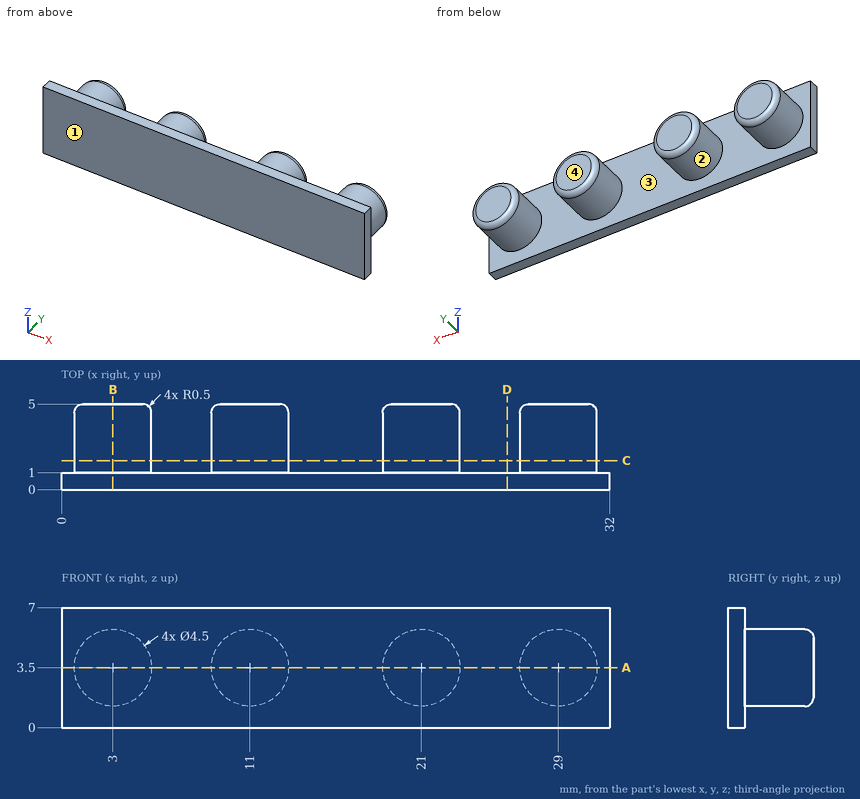
Answer from the drawing. Dimensions are ordinates in mm from the lowest x, y and z of the part. A direction names the side the tool comes from. Give positions to 0.01 mm unless a question says otherwise; leave off trailing zeros. Loops run counter-clockwise (first coordinate to the right, second up) from the corner with the lowest first, then second, coordinate; pieces in that order, holes last.
Item 1: Find the intervals of material crossed by line 1 along X through (y, z) = (2.4, 3.5); line 2 along X through (y, z) = (4.6, 5.5); line 3 along Y through (x, z) = (24, 4), in increasing order.
Item 2: The part is cut by section A-A (z = 3.5). Write down the section's boundary in (x, y), and give its area (3 significant figures).
Item 3: The part is cut by section C-C (y = 1.7). Write down the section's boundary in (x, z).
Item 4: Each of these flat-tipped pins is pushed along its axis until it touches: pin 1 Ø1.5 at (y, z) = (2.5, 2) entering from +X; pin 2 Ø1 at (y, z) = (3.5, 1) entering from +X. Where does it stop, or does it pass through?
Item 5: The mould has two halves that part along X. Classify the marked faces 3 and 4: released by +X, released by -X, zero draft, split by the parting line, or undercut.
Item 6: The part is cut by section B-B (x = 3). Write down the section's boundary in (y, z), and give its area (3 significant figures).
Item 7: For the marked faces 1 and 2, determine the directions among +Z, -Z, +X, -X, +Y, -Y from which every point of the face is accessible in a straight line to the end or side of a thin tool.
Item 8: The part is cut by section D-D (x = 26). Write down the section's boundary in (y, z), and give its area (3 significant figures).
Taken from the geometry:
1. line 1: x = 0.75 to 5.25, 8.75 to 13.25, 18.75 to 23.25, 26.75 to 31.25
1. line 2: x = 1.99 to 4.01, 9.99 to 12.01, 19.99 to 22.01, 27.99 to 30.01
1. line 3: y = 0 to 1
2. outline: (0, 0) - (32, 0) - (32, 1) - (31.25, 1) - (31.25, 4.5) arc R0.5 ccw to (30.75, 5) - (27.25, 5) arc R0.5 ccw to (26.75, 4.5) - (26.75, 1) - (23.25, 1) - (23.25, 4.5) arc R0.5 ccw to (22.75, 5) - (19.25, 5) arc R0.5 ccw to (18.75, 4.5) - (18.75, 1) - (13.25, 1) - (13.25, 4.5) arc R0.5 ccw to (12.75, 5) - (9.25, 5) arc R0.5 ccw to (8.75, 4.5) - (8.75, 1) - (5.25, 1) - (5.25, 4.5) arc R0.5 ccw to (4.75, 5) - (1.25, 5) arc R0.5 ccw to (0.75, 4.5) - (0.75, 1) - (0, 1) - close
2. area: 104 mm2
3. outline: circle Ø4.5 at (3, 3.5); circle Ø4.5 at (11, 3.5); circle Ø4.5 at (21, 3.5); circle Ø4.5 at (29, 3.5)
4. pin 1: stops at x = 31.12
4. pin 2: stops at x = 30.03
5. face 3: undercut
5. face 4: zero draft
6. outline: (0, 0) - (1, 0) - (1, 1.25) - (4.5, 1.25) arc R0.5 ccw to (5, 1.75) - (5, 5.25) arc R0.5 ccw to (4.5, 5.75) - (1, 5.75) - (1, 7) - (0, 7) - close
6. area: 24.9 mm2
7. face 1: +Z, -Z, +X, -X, -Y
7. face 2: +Y
8. outline: (0, 0) - (1, 0) - (1, 7) - (0, 7) - close
8. area: 7.00 mm2
